Verification items for the finished model (mm, model axes). A direction names the side the tool comes from. Coordinates: 2 decimals unless noted, no trailing zeros. Order: outer loops, then holes, each group sorted by start corner. A loop starts at its lowest first (then second) coordinate and runs counter-clockwise, first axis right, second up. Notation, with made-up numbers: (-7, 87) -> (41, 87) arc R12 cw to (41, 100) -> close; hole circle Ø3 at (89, 89.25). An arc over 180 degrees is marked (long way). Write each question's results on one line, items separated by ' | '. Start each with the question number.
(1) Cross-section at A-A on z = 12. Enter the section's corners in (x, y).
(2) Cross-section at B-B on x = 7. Enter the section's corners in (y, z).
(3) Set-up check for faces 1 (the flat face through (12, -12, 24.5)), 2 (the flat face through (-12, 0.5, 12)), 3 (the flat face through (24.5, -12, 12)): record each of +Z, -Z, +X, -X, +Y, -Y from which the full face is reachable in a straight line by a thin tool's end or side.
(4) Go/stop test with flat-tipped pins: pin 1 (12 mm diameter, centred on y = -15.5, z = 14, fed in from +X); pin 2 (19 mm diameter, centred on x = -15.5, y = 11, fed in from -Z); pin 3 (7 mm diameter, centred on x = -10.5, z = 16, fed in from -Y). Record where each tip stops, or that it passes through.
(5) Thickness scan on probe 1 along Y at (x, z) = (-10, 23). Record the ranges inside material, lowest first. Write a range as [from, to].
(6) Cross-section at C-C on y = -14. Enter the section's corners in (x, z), and give its area (3 significant figures).
```python
from build123d import *

# Parameters (mm, degrees)
F0_W     = 25
F0_H     = 25
F1_DEPTH = 25
F2_W     = 24
F2_H     = 24
F3_DEPTH = 25
F4_W     = 24
F4_H     = 24
F5_DEPTH = 25
F6_W     = 24
F6_H     = 24
F7_DEPTH = 25


with BuildPart() as f1:
    # F0 (on Right) → F1 (new body)
    with BuildSketch(Plane.YZ):
        with Locations((12.5, 12.5)):
            Rectangle(F0_W, F0_H)
    extrude(amount=F1_DEPTH)

    # F2 (on Right) → F3 (join)
    with BuildSketch(Plane.YZ):
        with Locations((12.5, 12.5)):
            Rectangle(F2_W, F2_H)
    extrude(amount=-F3_DEPTH)

    # F4 (on face) → F5 (join)
    with BuildSketch(Plane.XZ):
        with Locations((12.5, 12.5)):
            Rectangle(F4_W, F4_H)
    extrude(amount=F5_DEPTH)

    # F6 (on face) → F7 (join)
    with BuildSketch(Plane.XY.offset(25)):
        with Locations((12.5, 12.5)):
            Rectangle(F6_W, F6_H)
    extrude(amount=F7_DEPTH)


solid = f1.part
```
Results are:
1) outline: (-25, 0.5) -> (0, 0.5) -> (0, 0) -> (0.5, 0) -> (0.5, -25) -> (24.5, -25) -> (24.5, 0) -> (25, 0) -> (25, 25) -> (0, 25) -> (0, 24.5) -> (-25, 24.5) -> close
2) outline: (-25, 0.5) -> (0, 0.5) -> (0, 0) -> (25, 0) -> (25, 25) -> (24.5, 25) -> (24.5, 50) -> (0.5, 50) -> (0.5, 25) -> (0, 25) -> (0, 24.5) -> (-25, 24.5) -> close
3) face 1: +Z, +X, -X, -Y | face 2: +Z, -Z, -X, -Y | face 3: +Z, -Z, +X, -Y
4) pin 1: stops at x = 24.5 | pin 2: stops at z = 0.5 | pin 3: stops at y = 0.5
5) probe 1: y = [0.5, 24.5]
6) outline: (0.5, 0.5) -> (24.5, 0.5) -> (24.5, 24.5) -> (0.5, 24.5) -> close | area: 576 mm2
